from build123d import *

# Parameters (mm, degrees)
BOSS_EXTRUDE1_DEPTH = 6.35
SKETCH2_R           = 5.55625
BOSS_EXTRUDE2_DEPTH = 4
SKETCH4_R           = 4.805
BOSS_EXTRUDE3_DEPTH = 4
SKETCH5_R           = 5.55625
BOSS_EXTRUDE4_DEPTH = 4
SKETCH6_R           = 4.805
BOSS_EXTRUDE5_DEPTH = 4
FILLET1_R           = 5


with BuildPart() as part:
    # Sketch1 → Boss-Extrude1 (new body)
    with BuildSketch(Plane(origin=(0, 0, 0), x_dir=(1, 0, 0), z_dir=(0, 1, 0))):
        with BuildLine():
            Line((0, 9.539392014), (0, 0))
            Line((0, 0), (6, 0))
            Line((6, 0), (6, 9.539392014))
            ThreePointArc((6, 9.539392014), (3, 10), (0, 9.539392014))
        make_face()
        with BuildLine():
            Line((6, 0), (0, 0))
            Line((0, 0), (0, 9.539392014))
            ThreePointArc((0, 9.539392014), (-2.916079783, -8.062257748), (13, 0))
            ThreePointArc((13, 0), (11.062257748, 5.916079783), (6, 9.539392014))
            Line((6, 9.539392014), (6, 0))
        make_face()
        with BuildLine():
            Line((0, 142.860607986), (0, 9.539392014))
            ThreePointArc((0, 9.539392014), (3, 10), (6, 9.539392014))
            Line((6, 9.539392014), (6, 142.860607986))
            ThreePointArc((6, 142.860607986), (3, 142.4), (0, 142.860607986))
        make_face()
        with BuildLine():
            ThreePointArc((13, 152.4), (-2.916079783, 160.462257748), (0, 142.860607986))
            Line((0, 142.860607986), (0, 152.4))
            Line((0, 152.4), (6, 152.4))
            Line((6, 152.4), (6, 142.860607986))
            ThreePointArc((6, 142.860607986), (11.062257748, 146.483920217), (13, 152.4))
        make_face()
        with BuildLine():
            Line((0, 152.4), (0, 142.860607986))
            ThreePointArc((0, 142.860607986), (3, 142.4), (6, 142.860607986))
            Line((6, 142.860607986), (6, 152.4))
            Line((6, 152.4), (0, 152.4))
        make_face()
    extrude(amount=BOSS_EXTRUDE1_DEPTH)

    # Sketch2 → Boss-Extrude2 (add)
    with BuildSketch(Plane(origin=(0, 6.35, 0), x_dir=(1, 0, 0), z_dir=(0, 1, 0))):
        with Locations(Location((3, 152.4, 0), (0, 0, 270))):
            Circle(SKETCH2_R)
    extrude(amount=BOSS_EXTRUDE2_DEPTH)

    # Sketch4 → Boss-Extrude3 (add)
    with BuildSketch(Plane(origin=(0, 10.35, 0), x_dir=(1, 0, 0), z_dir=(0, 1, 0))):
        with Locations(Location((3, 152.4, 0), (0, 0, 270))):
            Circle(SKETCH4_R)
    extrude(amount=BOSS_EXTRUDE3_DEPTH)

    # Sketch5 → Boss-Extrude4 (add)
    with BuildSketch(Plane.XZ):
        with Locations(Location((3, 0, 0), (0, 0, 270))):
            Circle(SKETCH5_R)
    extrude(amount=BOSS_EXTRUDE4_DEPTH)

    # Sketch6 → Boss-Extrude5 (add)
    with BuildSketch(Plane.XZ.offset(4)):
        with Locations(Location((3, 0, 0), (0, 0, 270))):
            Circle(SKETCH6_R)
    extrude(amount=BOSS_EXTRUDE5_DEPTH)

    # Fillet1
    fillet1_edges = [part.edges().sort_by_distance(p)[0] for p in [
        (0, 3.175, -9.539392014),
        (0, 3.175, -142.860607986),
        (6, 3.175, -142.860607986),
        (6, 3.175, -9.539392014),
    ]]
    fillet(fillet1_edges, radius=FILLET1_R)


solid = part.part
The listing builds one solid part. Answer for the finished solid, in the listing's coordinates (mm). A direction names the side the tool comes from. Give positions to 0.01 mm unless a question says otherwise; leave off trailing zeros. Write each loop counter-clockwise with the first axis right and the second up, starting at its lowest first coordinate (ties: lowest second). Pieces come first, ordered by that corner, then holes. Notation, with made-up numbers: (9.5, -25) -> (36.5, -25) arc R23 cw to (36.5, -7) -> close; hole circle Ø6 at (23, 68.25). An arc over 180 degrees is marked (long way). One line per question, with ' | ' between items. Start each with the question number.
1. For faces 4 (the cylindrical face through (6.605, 3.219, -142.096)), 5 (the flat face through (3, 14.35, -152)), 6 (the cylindrical face through (4.443, -5.972, -4.583)), 7 (the cylindrical face through (1.16, 12.32, -147.96)), 8 (the cylindrical face through (-0.64, 3.22, -10.24)), determine the directions among +Z, -Z, +X, -X, +Y, -Y from which every point of the face is accessible in a straight line to the end or side of a thin tool.
2. Section C-C (y = 12) is taken. Determine the outline of the cut face in (x, z) (3 decimals), plus the area to 3 significant figures.
3. Section D-D (z = -10) is taken. Determine the outline of the cut face in (x, y).
4. Find the intervals of material crossed by probe 1 along Y at (x, z) = (0.75, -40); probe 2 along X at (y, z) = (3.75, -51); probe 3 along Z at (x, y) = (8, 3), in increasing order.
5. Section A-A (x = 3) is taken. Determine the outline of the cut face in (y, z) (3 decimals), plus the area to 3 significant figures.
6. Section B-B (z = -29.5) is taken. Determine the outline of the cut face in (x, y).
7. For a pull along Z with two mould halves and no side action, classify faces 1 (the flat face through (8, 10.35, -154)), 2 (the cylindrical face through (4.67, 8.32, -147.1)), 3 (the flat face through (6, 3, -75)) as pulls with the +Z half, pulls with the -Z half, needs draft (parallel to the pull), parting line crosses it, or undercut.
8. Given pin 1 Ø4 at (y, z) = (-3, -44) entering from -X; pin 2 Ø5 at (x, y) = (2.5, -4) entering from +Z; pin 3 Ø6 at (x, z) = (3, -68) entering from +Y; pin 4 Ø3 at (y, z) = (1.5, -101.5) entering from -X, each flat-ended and moving along its own axis, determine where each tip first touches the part or whether it passes through.
Response values:
1) face 4: +X, +Y, -Y | face 5: +Z, -Z, +X, -X, +Y | face 6: -Y | face 7: +Y | face 8: -X, +Y, -Y
2) outline: circle Ø9.61 at (3, -152.4) | area: 72.5 mm2
3) outline: (-0.78, 0) -> (6.78, 0) -> (6.78, 6.35) -> (-0.78, 6.35) -> close
4) probe 1: 0 to 6.35 | probe 2: 0 to 6 | probe 3: -161.06 to -143.71, -8.69 to 8.66
5) outline: (-8, -4.805) -> (-4, -4.805) -> (-4, -5.556) -> (0, -5.556) -> (0, -162.4) -> (6.35, -162.4) -> (6.35, -157.956) -> (10.35, -157.956) -> (10.35, -157.205) -> (14.35, -157.205) -> (14.35, -147.595) -> (10.35, -147.595) -> (10.35, -146.844) -> (6.35, -146.844) -> (6.35, 10) -> (0, 10) -> (0, 5.556) -> (-4, 5.556) -> (-4, 4.805) -> (-8, 4.805) -> close | area: 1,260 mm2
6) outline: (0, 0) -> (6, 0) -> (6, 6.35) -> (0, 6.35) -> close
7) face 1: needs draft | face 2: parting line crosses it | face 3: undercut
8) pin 1: through | pin 2: z = 5.56 | pin 3: y = 6.35 | pin 4: x = 0
